Here's the drawing with two shaded views (mm, measured from the low corner). I have some questions. A direction names the side the tool comes from. Coordinates: 2 decimals unless noted, no trailing zeros. Order: outer loops, then holes, each group sorted by start corner. A loop starts at its lowest first (then second) coordinate and runs counter-clockwise, first axis right, second up. Notation, with made-up numbers: (-17, 65.25) -> (-10, 65.25) arc R29 cw to (-10, 100.25) -> close; hole circle Ø4 at (1, -33). An arc over 180 degrees is marked (long way). Write item = value, one per line.
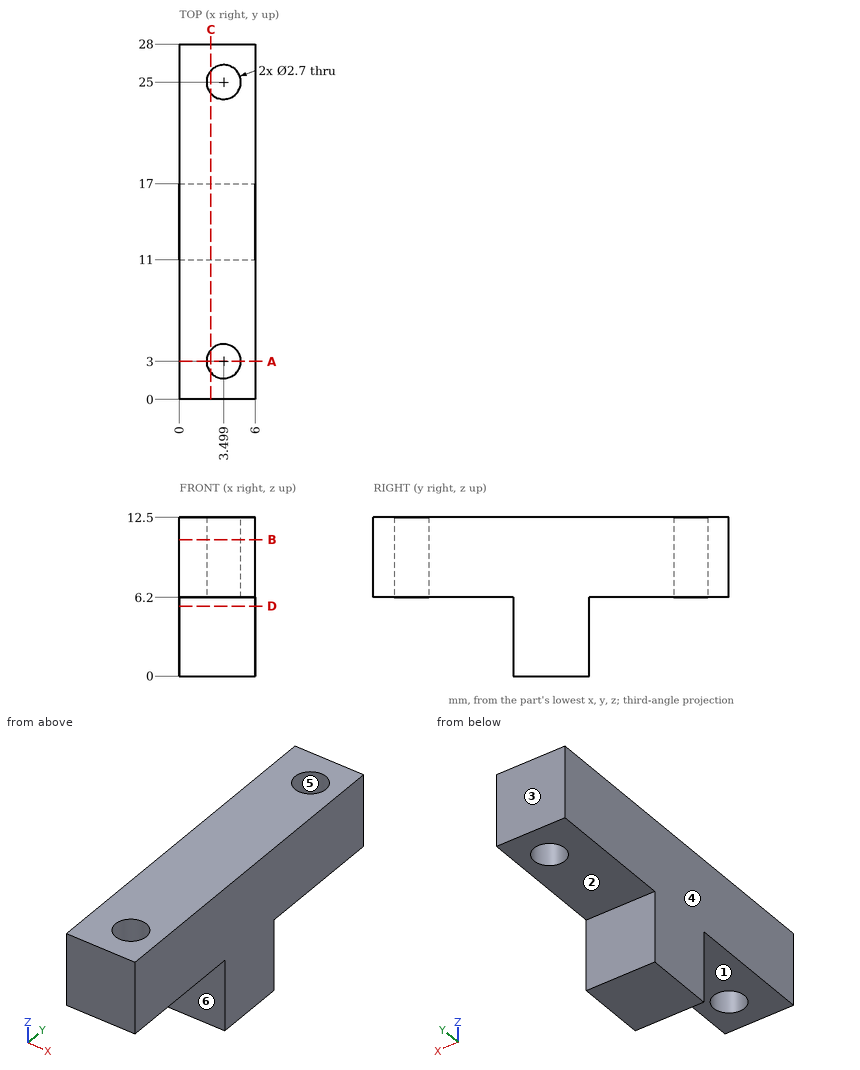
Item 1: I want a section at C-C, the plane x = 2.5. Please give me the cut outline in (y, z).
A:
outline = (0, 6.2) -> (2.09, 6.2) -> (2.09, 12.5) -> (0, 12.5) -> close; (3.91, 6.2) -> (11, 6.2) -> (11, 0) -> (17, 0) -> (17, 6.2) -> (24.09, 6.2) -> (24.09, 12.5) -> (3.91, 12.5) -> close; (25.91, 6.2) -> (28, 6.2) -> (28, 12.5) -> (25.91, 12.5) -> close
Item 2: If we mould it in two halves opening along X, with no side actions, what happens to the marked faces 4, 5 and 6? For each: pulls with the +X half, pulls with the -X half, needs draft (parallel to the pull), parting line crosses it, or undercut.
A:
face_4 = pulls with the -X half
face_5 = undercut
face_6 = needs draft
Item 3: I'm going to push flat-ended pins straight in: P1, Ø1.6, axis at x = 3.5, y = 25, coming from the +Z side; P2, Ø3, axis at x = 1.5, y = 5, coming from the -Z side; P3, Ø1.5, axis at x = 3, z = 4.5, coming from the +Y side; P4, Ø1, axis at x = 4.5, z = 1.5, coming from the -Y side. Where does each tip first touch, or does it pass through?
A:
P1 = through
P2 = 6.2
P3 = 17
P4 = 11
Item 4: If I drill on probe 1 along Y at (x, z) = (3.5, 9.5); probe 2 along Z at (x, y) = (0.75, 7.75); probe 3 along Y at (x, z) = (5.5, 6), over which ranges is the centre line in solid material (lowest first)?
A:
probe_1 = 0 to 1.65, 4.35 to 23.65, 26.35 to 28
probe_2 = 6.2 to 12.5
probe_3 = 11 to 17
Item 5: I want a section at B-B, the plane z = 10.75. Please give me the cut outline in (x, y).
A:
outline = (0, 0) -> (6, 0) -> (6, 28) -> (0, 28) -> close; hole circle Ø2.7 at (3.5, 3); hole circle Ø2.7 at (3.5, 25)
Item 6: I want a section at D-D, the plane z = 5.5. Please give me the cut outline in (x, y), plus the area to 3 significant figures.
A:
outline = (0, 11) -> (6, 11) -> (6, 17) -> (0, 17) -> close
area = 36.0 mm2
Item 7: For the marked faces 1, 2 and 3, which set-ups out of +Z, -Z, +X, -X, +Y, -Y let a thin tool reach every point of the face, with its end or its side?
A:
face_1 = -Z, +X, -X, -Y
face_2 = -Z, +X, -X, +Y
face_3 = +Z, -Z, +X, -X, +Y
Item 8: I want a section at A-A, the plane y = 3. Please give me the cut outline in (x, z).
A:
outline = (0, 6.2) -> (2.15, 6.2) -> (2.15, 12.5) -> (0, 12.5) -> close; (4.85, 6.2) -> (6, 6.2) -> (6, 12.5) -> (4.85, 12.5) -> close
